Verification items for the finished model (mm, model axes). Face numbers are marked on the shaded views. A direction names the side the tool comes from. Give positions to 0.01 mm unless a question says otherwise; leave off trailing zeros. Loops run counter-clockwise (first coordinate to the right, second up) from the corner with the lowest first, then second, coordinate; pieces in that order, holes last. Notation, with made-up numbers: (8, 82.25) - (26, 82.25) arc R33 cw to (26, 112.25) - close; hole circle Ø6 at (32, 44.25). An arc over 180 degrees is marked (long way). Use one line per item in the form item = value.
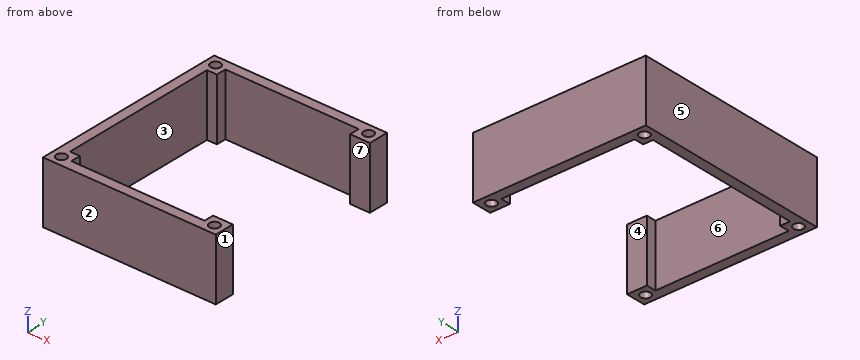
Autodesk Inventor part; units mm, degrees
ref_plane "YZ Plane" through (0, 0, 0) normal (1, 0, 0) x (0, 1, 0)
ref_plane "XZ Plane" through (0, 0, 0) normal (0, 1, 0) x (-1, 0, 0)
ref_plane "XY Plane" through (0, 0, 0) normal (0, 0, 1) x (1, 0, 0)
sketch "Sketch1" plane through (0, 0, 0) normal (0, 0, 1) x (1, 0, 0)
  line L0 (0, 0) -> (0, 101.6)
  line L1 (0, 101.6) -> (88.9, 101.6)
  line L2 (0, 0) -> (88.9, 0)
  arc A0 (88.9, 0) -> (88.9, 101.6) centre (-27.4974, 50.8) ccw
  line L3 (0, 101.6) -> (5.08, 101.6) construction
  line L4 (5.08, 101.6) -> (5.08, 96.52) construction
  circle A1 centre (5.08, 96.52) radius 2.5797
  line L5 (44.45, 101.6) -> (44.45, 0) construction
  line L6 (0, 50.8) -> (104.3223, 50.8) construction
  circle A2 centre (83.82, 96.52) radius 2.5797
  circle A3 centre (5.08, 5.08) radius 2.5797
  circle A4 centre (83.82, 5.08) radius 2.5797
  line L7 (0, 101.6) -> (10.16, 101.6) construction
  line L8 (0, 101.6) -> (0, 91.44) construction
  line L9 (10.16, 96.52) -> (10.16, 91.44)
  line L10 (10.16, 91.44) -> (5.08, 91.44)
  line L11 (5.08, 91.44) -> (5.08, 50.8)
  line L12 (10.16, 96.52) -> (44.45, 96.52)
  arc A5 (90.1405, 10.16) -> (90.1405, 91.44) centre (-27.4974, 50.8) ccw
  line L13 (84.2708, 99.06) -> (83.3692, 99.06)
  line L14 (78.74, 96.52) -> (78.74, 91.44)
  line L15 (78.74, 91.44) -> (90.1405, 91.44)
  line L16 (78.74, 96.52) -> (44.45, 96.52)
  line L17 (10.16, 5.08) -> (10.16, 10.16)
  line L18 (10.16, 10.16) -> (5.08, 10.16)
  line L19 (10.16, 5.08) -> (44.45, 5.08)
  line L20 (78.74, 5.08) -> (44.45, 5.08)
  line L21 (78.74, 5.08) -> (78.74, 10.16)
  line L22 (78.74, 10.16) -> (90.1405, 10.16)
  line L23 (5.08, 10.16) -> (5.08, 50.8)
  point P0 (78.74, 101.6)
  point P1 (88.9, 91.44)
  point P2 (10.16, 0)
  point P3 (0, 10.16)
  point P4 (78.74, 0)
  point P5 (88.9, 10.16)
  dimension "d0" = 101.6
  dimension "d1" = 88.9
  dimension "d2" = 88.9
  dimension "d3" = 127
  dimension "d4" = 5.08
  dimension "d5" = 5.08
  dimension "d6" = 5.1594
  dimension "d7" = 10.16
  dimension "d8" = 10.16
  dimension "d9" = 2.54
extrude "Extrusion1" add sketch "Sketch1" along normal blind 31.6992
sketch "Sketch2" plane through (0, 0, 31.6992) normal (0, 0, 1) x (1, 0, 0)
  line L0 (88.9, 0) -> (0, 0)
  line L1 (88.9, 0) -> (124.549, 0)
  line L2 (124.549, 0) -> (124.549, 101.6)
  line L3 (124.549, 101.6) -> (88.9, 101.6)
  line L4 (88.9, 101.6) -> (88.9, 0)
extrude "Extrusion2" cut sketch "Sketch2" against normal blind 31.6992
properties part number "Gearbox cover"
1. Depth check by flat-ended pin: pin 1 Ø3 at (x, y) = (5.08, 5.08) entering from -Z; pin 2 Ø12 at (y, z) = (36, 11) entering from +X. Enter the tip coordinate at first touch or a pass-through.
Result set:
pin_1 = through
pin_2 = 5.08
2. Section check C-C, the plane x = 38. Record the cut outline in (y, z).
Result set:
outline = (0, 0) - (5.08, 0) - (5.08, 31.7) - (0, 31.7) - close; (96.52, 0) - (101.6, 0) - (101.6, 31.7) - (96.52, 31.7) - close
3. Scan lines: probe 1 along Y at (x, z) = (83.82, 16); probe 2 along Y at (x, z) = (5, 23.5); probe 3 along Y at (x, z) = (69, 25.5). Record each from-to range of solid material in increasing order.
Result set:
probe_1 = 0 to 2.5, 7.66 to 10.16, 91.44 to 93.94, 99.1 to 101.6
probe_2 = 0 to 2.5, 7.66 to 93.94, 99.1 to 101.6
probe_3 = 0 to 5.08, 96.52 to 101.6
4. Tool access check on the marked faces 5, 6 and 7. Record the directions out of +Z, -Z, +X, -X, +Y, -Y that give a thin tool (end or side, any length) a straight path to the whole face; none if there is none.
Result set:
face_5 = +Z, -Z, -X, +Y, -Y
face_6 = +Z, -Z
face_7 = +Z, -Z, +X
5. Section check D-D, the plane y = 34.5. Record the cut outline in (x, z), then the cut area to 3 significant figures.
Result set:
outline = (0, 0) - (5.08, 0) - (5.08, 31.7) - (0, 31.7) - close
area = 161 mm²
6. Section check A-A, the plane x = 83.82. Record the cut outline in (y, z), then the cut area to 3 significant figures.
Result set:
outline = (0, 0) - (2.5, 0) - (2.5, 31.7) - (0, 31.7) - close; (7.66, 0) - (10.16, 0) - (10.16, 31.7) - (7.66, 31.7) - close; (91.44, 0) - (93.94, 0) - (93.94, 31.7) - (91.44, 31.7) - close; (99.1, 0) - (101.6, 0) - (101.6, 31.7) - (99.1, 31.7) - close
area = 317 mm²
7. Draft check along Y on the marked faces 1, 2, 3 and 4. Enter one of: released by +Y, released by -Y, zero draft, split by the parting line, or undercut.
Result set:
face_1 = zero draft
face_2 = released by -Y
face_3 = undercut
face_4 = undercut
8. Section check B-B, the plane z = 12. Record the cut outline in (x, y), then the cut area to 3 significant figures.
Result set:
outline = (0, 0) - (88.9, 0) - (88.9, 10.16) - (78.74, 10.16) - (78.74, 5.08) - (10.16, 5.08) - (10.16, 10.16) - (5.08, 10.16) - (5.08, 91.44) - (10.16, 91.44) - (10.16, 96.52) - (78.74, 96.52) - (78.74, 91.44) - (88.9, 91.44) - (88.9, 101.6) - (0, 101.6) - close; hole circle Ø5.16 at (5.08, 5.08); hole circle Ø5.16 at (5.08, 96.52); hole circle Ø5.16 at (83.82, 5.08); hole circle Ø5.16 at (83.82, 96.52)
area = 1,440 mm²
